Check sheet for the modelled part. Datum: model origin and axes. Units: mm. Round coordinates to 2 decimals unless told otherwise and drop trailing zeros. Order: outer loops, then holes, each group sorted by start corner. A loop starts at its lowest first (then second) coordinate and runs counter-clockwise, first axis right, second up.
(1) Mould release check, pull along Z, two halves, no side actions. Record for faces 1 (the flat face through (130, 9, 5)), 2 (the cylindrical face through (6.161, 9.126, 6.064)), 3 (the flat face through (64, 9, 0)), 4 (the flat face through (64, 9, 10)): released by +Z, released by -Z, zero draft, split by the parting line, or undercut.
(2) Sectioned sample at B-B, the plane x = 5. Enter the section's corners in (y, z) (3 decimals).
(3) Thickness scan on probe 1 along Z at (x, y) = (5, 13.5) (3 decimals); probe 2 along X at (y, z) = (14, 5.25). Record the ranges inside material, lowest first.
(4) Sectioned sample at A-A, the plane z = 5. Enter the section's corners in (x, y) (3 decimals), and give its area (3 significant figures).
```python
from build123d import *

# Parameters (mm, degrees)
F0_W     = 130
F0_H     = 18
F1_DEPTH = 10
F3_D     = 3.15


with BuildPart() as f1:
    # F0 (on Top) → F1 (new body)
    with BuildSketch(Plane.XY):
        with Locations((65, 9)):
            Rectangle(F0_W, F0_H)
    extrude(amount=F1_DEPTH)

    # F3 (through all)
    with Locations(Plane.XZ):
        with Locations((5, 5)):
            Hole(F3_D / 2)


solid = f1.part
```
Derived:
1. face 1: zero draft
1. face 2: undercut
1. face 3: released by -Z
1. face 4: released by +Z
2. outline: (0, 0) - (18, 0) - (18, 3.425) - (0, 3.425) - close; (0, 6.575) - (18, 6.575) - (18, 10) - (0, 10) - close
3. probe 1: z = 0 to 3.425, 6.575 to 10
3. probe 2: x = 0 to 3.44, 6.56 to 130
4. outline: (0, 0) - (3.425, 0) - (3.425, 18) - (0, 18) - close; (6.575, 0) - (130, 0) - (130, 18) - (6.575, 18) - close
4. area: 2,280 mm2
